Input: part model. Units: mm. Frame: model coordinates. Give positions to 0.01 mm unless a question says otherwise; leave off trailing zeros. Loops run counter-clockwise (first coordinate to the right, second up) from the corner with the lowest first, then second, coordinate; pieces in that order, holes last. Notation, with made-up numbers: M 41,50 L 78,50 A30 cw 78,79 Z; hole C 38.25,55 d2. An arc over 180 degrees is marked long. Answer as a JSON object with one key per item and string values. Group by question number.
1) Ray query, L1, parallel to X at y = -3.4, z = -12.5; L2, parallel to X at y = -0.6, z = 16; L3, parallel to X at y = -1.05, z = -45.5. Return the intervals inside material, ascending.
2) Section query C-C on x = -169. Return loops of the section in (y, z).
3) Section query A-A on y = -2.9. Return loops of the section in (x, z).
4) Section query B-B on z = 1.5. Return loops of the section in (x, y).
5) Draft query along X for faces 1 (the cylindrical face through (96.079, -2.028, -24.855)), 2 (the flat face through (-197.211, -1.972, -56.153)), 3 (the flat face through (101, 0, -31)). Return one class per face: +X half, -X half, draft (parallel to the pull), parting line (faces both ways), or undercut.
6) First-contact query: P1, Ø1.5, axis at x = 223, y = -2, coming from the +Z side; P2, Ø1.5, axis at x = -28, y = -2.5, coming from the +Z side; P3, Ø2, axis at y = -1.5, z = 3, coming from the -X side. Flat tips, straight axial feed; report the tip coordinate or a pass-through.
from build123d import *

# Parameters (mm, degrees)
F1_DEPTH = 4
F2_SIZE  = 20
F3_R     = 5
F4_DEPTH = 25
F5_R     = 4.25
F6_DEPTH = 25


with BuildPart() as f1:
    # F0 (on Front) → F1 (new body)
    with BuildSketch(Plane.XZ):
        Polygon((92.662452, -21.205135), (-207.337548, -21.205135), (-207.337548, -65.482802), (92.662452, -81.205135), align=None)
        Polygon((92.662452, 28.794865), (92.662452, -21.205135), (92.662452, -81.205135), (302.662452, -92.210769), (302.662452, 17.789231), align=None)
    extrude(amount=F1_DEPTH)

    # F2
    f2_edges = [f1.edges().sort_by_distance(p)[0] for p in [
        (-207.337548, -2, -65.482802),
    ]]
    chamfer(f2_edges, length=F2_SIZE)

    # F3 (on face) → F4 (cut)
    with BuildSketch(Plane.XZ.offset(4)):
        with Locations((92.662452, -21.205135)):
            Circle(F3_R)
    extrude(amount=-F4_DEPTH, mode=Mode.SUBTRACT)

    # F5 (on face) → F6 (cut)
    with BuildSketch(Plane.XZ.offset(4)):
        with Locations((277.662452, -12.210769)):
            Circle(F5_R)
        with Locations((277.662452, -62.210769)):
            Circle(F5_R)
    extrude(amount=-F6_DEPTH, mode=Mode.SUBTRACT)


solid = f1.part
Output:
{
 "1": {"L1": "x = 92.66 to 273.42, 281.9 to 302.66", "L2": "x = 92.66 to 302.66", "L3": "x = -207.32 to 302.66"},
 "2": {"outline": "M -4,-67.49 L 0,-67.49 L 0,-21.21 L -4,-21.21 Z"},
 "3": {"outline": "M -207.34,-45.48 L -187.36,-66.53 L 302.66,-92.21 L 302.66,17.79 L 92.66,28.79 L 92.66,-16.21 A5 cw long 87.66,-21.21 L -207.34,-21.21 Z; hole C 277.66,-62.21 d8.5; hole C 277.66,-12.21 d8.5"},
 "4": {"outline": "M 92.66,-4 L 302.66,-4 L 302.66,0 L 92.66,0 Z"},
 "5": {"face 1": "undercut", "face 2": "-X half", "face 3": "draft"},
 "6": {"P1": "stops at z = 22", "P2": "stops at z = -21.21", "P3": "stops at x = 92.66"}
}
